```python
from build123d import *

# Parameters (mm, degrees)
SKIZZE2_R                       = 5
SKIZZE2_R_2                     = 4
AUFSATZ_LINEAR_AUSTRAGEN1_DEPTH = 1
SKIZZE2_2_R                     = 4
AUFSATZ_LINEAR_AUSTRAGEN2_DEPTH = 35
M4_GEWINDEBOHRUNG1_D            = 3.3
M4_GEWINDEBOHRUNG1_DEPTH        = 10
M4_GEWINDEBOHRUNG1_TIP          = 0.991420021
SCHNITT_LINEAR_AUSTRAGEN1_DEPTH = 1.5
SKIZZE7_W                       = 8
SKIZZE7_H                       = 3.641356754
SCHNITT_LINEAR_AUSTRAGEN2_DEPTH = 29
FASE1_SIZE                      = 0.5


with BuildPart() as part:
    # Skizze1 → Rotation1 (revolve)
    with BuildSketch(Plane.XY):
        Polygon((27.5, 0), (-27.5, 0), (-27.5, 24.349478444), (-21.5, 31.5), (19.5, 31.5), (27.5, 26.881197846), align=None)
    revolve(axis=Axis((27.5, 0, 0), (-1, 0, 0)))

    # Skizze2 → Aufsatz-Linear austragen1 (add)
    with BuildSketch(Plane(origin=(27.5, 0, 0), x_dir=(0, 0, -1), z_dir=(1, 0, 0))):
        with Locations(Location((0, 0, 0), (0, 0, 90))):
            Circle(SKIZZE2_R)
        with Locations(Location((0, 0, 0), (0, 0, 90))):
            Circle(SKIZZE2_R_2, mode=Mode.SUBTRACT)
    extrude(amount=AUFSATZ_LINEAR_AUSTRAGEN1_DEPTH)

    # Skizze2<2> → Aufsatz-Linear austragen2 (add)
    with BuildSketch(Plane(origin=(27.5, 0, 0), x_dir=(0, 0, -1), z_dir=(1, 0, 0))):
        with Locations(Location((0, 0, 0), (0, 0, 90))):
            Circle(SKIZZE2_2_R)
    extrude(amount=AUFSATZ_LINEAR_AUSTRAGEN2_DEPTH)

    # M4 Gewindebohrung1
    with Locations(Plane(origin=(27.5, 0, 0), x_dir=(0, 0, -1), z_dir=(1, 0, 0))):
        with Locations((0, 22), (0, -22), (22, 0), (-22, 0)):
            Hole(M4_GEWINDEBOHRUNG1_D / 2, depth=M4_GEWINDEBOHRUNG1_DEPTH)
            with Locations((0, 0, -(M4_GEWINDEBOHRUNG1_DEPTH + M4_GEWINDEBOHRUNG1_TIP / 2))):  # 118° drill point
                Cone(0, M4_GEWINDEBOHRUNG1_D / 2, M4_GEWINDEBOHRUNG1_TIP, mode=Mode.SUBTRACT)

    # Skizze6 → Schnitt-Linear austragen1 (cut)
    with BuildSketch(Plane.XY.offset(4)):
        with BuildLine():
            Line((37.00625, 1.50625), (53.99375, 1.50625))
            ThreePointArc((53.99375, 1.50625), (55.5, 0), (53.99375, -1.50625))
            Line((53.99375, -1.50625), (37.00625, -1.50625))
            ThreePointArc((37.00625, -1.50625), (35.5, 0), (37.00625, 1.50625))
        make_face()
    extrude(amount=-SCHNITT_LINEAR_AUSTRAGEN1_DEPTH, mode=Mode.SUBTRACT)

    # Skizze7 → Schnitt-Linear austragen2 (cut)
    with BuildSketch(Plane(origin=(62.5, 0, 0), x_dir=(0, 0, -1), z_dir=(1, 0, 0))):
        with Locations((0, 5.320678377)):
            Rectangle(SKIZZE7_W, SKIZZE7_H)
    extrude(amount=-SCHNITT_LINEAR_AUSTRAGEN2_DEPTH, mode=Mode.SUBTRACT)

    # Fase1
    fase1_edges = [part.edges().sort_by_distance(p)[0] for p in [
        (62.5, -4, 0),
    ]]
    chamfer(fase1_edges, length=FASE1_SIZE - 0.0001)  # a hair under: the kernel refuses the full size


solid = part.part
```
Here's how the part is built. I have some questions about the finished solid (model axes, mm). A direction names the side the tool comes from. Coordinates: 2 decimals unless noted, no trailing zeros. Loops run counter-clockwise (first coordinate to the right, second up) from the corner with the lowest first, then second, coordinate; pieces in that order, holes last. Notation, with made-up numbers: (-5, -17.75) - (13, -17.75) arc R26 cw to (13, 19.25) - close; hole circle Ø2 at (75.5, 33). An arc over 180 degrees is marked (long way). Answer as CSV lines item,"result".
Q1. We'd pull the mould along Y, two halves only. Please class faces 3 (the face through (46, 0, 2.5)), 4 (the face through (-27.125, 11.442, 21.999)), 5 (the face through (48, 3.5, 0)), 6 (the face through (62.5, 0, 0)): pulls with the +Y half, pulls with the -Y half, needs draft (parallel to the pull), parting line crosses it, or undercut.
Response:
face 3,"undercut"
face 4,"parting line crosses it"
face 5,"pulls with the +Y half"
face 6,"needs draft"
Q2. For pin 1 (1.5 mm diameter, centred on y = -23.5, z = 17, fed in from +X); pin 2 (3 mm diameter, centred on y = -22, z = 0, fed in from +X); pin 3 (5 mm diameter, centred on y = -19, z = 10, fed in from +X), each with a flat end and sliding along its axis, tell me the tip position at first contact or that it passes through.
Response:
pin 1,"x = 25.12"
pin 2,"x = 17.41"
pin 3,"x = 27.5"
Q3. If we section it at B-B, the plane x = -12: Write out the boundary of the cut face in (y, z), and give its area (3 significant figures).
Response:
outline,"circle Ø63 at (0, 0)"
area,"3,120 mm2"
Q4. If I drill on L1, parallel to Z at x = 22, y = 0; L2, parallel to Y at x = 25.75, z = 0; L3, parallel to Y at x = 20.5, z = 0, over which ranges is the centre line in solid material (lowest first)? Write a range as [from, to].
Response:
L1,"[-30.06, -23.65], [-20.35, 20.35], [23.65, 30.06]"
L2,"[-27.89, -23.65], [-20.35, 20.35], [23.65, 27.89]"
L3,"[-30.92, -23.65], [-20.35, 20.35], [23.65, 30.92]"
Q5. For faces 1 (the face through (-27.5, 0, 0)), 2 (the face through (22.43, 0.07, -23.65)), which set-ups out of +Z, -Z, +X, -X, +Y, -Y let a thin tool reach every point of the face, with its end or its side?
Response:
face 1,"+Z, -Z, -X, +Y, -Y"
face 2,"+X"
Q6. If we section it at A-A, the plane x = 46: Write out the boundary of the cut face in (y, z).
Response:
outline,"(-1.51, 2.5) - (-1.51, 3.71) arc R4 ccw (long way) to (3.5, -1.94) - (3.5, 1.94) arc R4 ccw to (1.51, 3.71) - (1.51, 2.5) - close"
